Autodesk Inventor part; units mm, degrees
ref_plane "YZ Plane" through (0, 0, 0) normal (1, 0, 0) x (0, 1, 0)
ref_plane "XZ Plane" through (0, 0, 0) normal (0, 1, 0) x (-1, 0, 0)
ref_plane "XY Plane" through (0, 0, 0) normal (0, 0, 1) x (1, 0, 0)
sketch "Sketch1" plane through (0, 0, 0) normal (0, 0, 1) x (1, 0, 0)
  line L0 (0, 0) -> (30, 0)
  line L1 (30, 0) -> (30, 12.5)
  line L2 (30, 12.5) -> (0, 12.5)
  line L3 (0, 12.5) -> (0, 0)
  circle A0 centre (15, 0) radius 8
  point P0 (7, 0)
  point P1 (23, 0)
  dimension "d0" = 30
  dimension "d1" = 12.5
  dimension "d2" = 16
extrude "Extrusion1" add sketch "Sketch1" along normal mid plane 16 contours A0 L0 L3 L2 L1
sketch "Sketch2" plane through (0, 12.5, 8) normal (0, 1, 0) x (1, 0, 0)
  line L0 (0, 16) -> (0, 0)
  line L1 (30, 0) -> (0, 0)
  line L2 (30, 16) -> (30, 0)
  line L3 (0, 16) -> (30, 16)
  line L4 (23, 0) -> (7, 0)
  line L5 (15, 0) -> (15, 16)
  line L6 (0, 8) -> (30, 8)
  line L7 (2.5, 3) -> (27.5, 3)
  line L8 (27.5, 3) -> (27.5, 13)
  line L9 (27.5, 13) -> (2.5, 13)
  line L10 (2.5, 13) -> (2.5, 3)
  point P0 (15, 8)
  dimension "d5" = 25
  dimension "d6" = 10
hole "Hole1" at (2.5, 12.5, 5) at (2.5, 12.5, -5) at (27.5, 12.5, -5) at (27.5, 12.5, 5) at (15, 12.5, 0) direction (0, -1, 0) diameter 3 end through all
fillet "Fillet1" radius 2 4 edges at (0, 6.25, 8) (30, 6.25, -8) (30, 6.25, 8) (0, 6.25, -8)
properties part number "base2" material "PVC-Piping"
Could you check a few things on this model? Use its own coordinates, in mm. Give positions to 0.01 mm unless a question says otherwise; leave off trailing zeros. Loops run counter-clockwise (first coordinate to the right, second up) from the corner with the lowest first, then second, coordinate; pieces in that order, holes last. Notation, with made-up numbers: M -8.75,70 L 11.25,70 A21 ccw 11.25,83 Z; hole C -3.75,-36.75 d2. An arc over 180 degrees is marked long. Answer as a JSON object with one key per item and string values.
Q1. If we mould it in two halves opening along X, with no side actions, what happens to faces 1 (the flat face through (3, 0, 0)), 2 (the cylindrical face through (0.57, 6.16, -7.4)), 3 (the cylindrical face through (26, 6, -5))? For each: pulls with the +X half, pulls with the -X half, needs draft (parallel to the pull), parting line crosses it, or undercut.
Values found:
{"face 1": "needs draft", "face 2": "pulls with the -X half", "face 3": "undercut"}
Q2. If I drill on probe 1 along Z at (x, y) = (27.5, 8); probe 2 along X at (y, z) = (5.25, -5); probe 3 along Z at (x, y) = (15, 9.3), over which ranges is the centre line in solid material (lowest first)? Write a range as [from, to].
Values found:
{"probe 1": "z = [-8, -6.5], [-3.5, 3.5], [6.5, 8]", "probe 2": "x = [0, 1], [4, 8.96], [21.04, 26], [29, 30]", "probe 3": "z = [-8, -1.5], [1.5, 8]"}
Q3. Suppose I cut it at C-C, the plane y = 4. List the corners of the cut face in (x, z) for me, plus the area to 3 significant figures.
Values found:
{"outline": "M 0,-6 A2 ccw 2,-8 L 8.07,-8 L 8.07,8 L 2,8 A2 ccw 0,6 Z; M 21.93,-8 L 28,-8 A2 ccw 30,-6 L 30,6 A2 ccw 28,8 L 21.93,8 Z; hole C 2.5,-5 d3; hole C 2.5,5 d3; hole C 27.5,-5 d3; hole C 27.5,5 d3", "area": "227 mm²"}
Q4. For P1, Ø2.5, axis at x = 2.5, z = 5, coming from the -Y side; P2, Ø4, axis at x = 18.5, z = -2, coming from the -Y side, each with a flat end and sliding along its axis, tell me the tip position at first contact or that it passes through.
Values found:
{"P1": "passes through", "P2": "stops at y = 5.81"}
Q5. Suppose I cut it at A-A, the plane x = 2.5. List the corners of the cut face in (y, z) for me.
Values found:
{"outline": "M 0,-8 L 12.5,-8 L 12.5,-6.5 L 0,-6.5 Z; M 0,-3.5 L 12.5,-3.5 L 12.5,3.5 L 0,3.5 Z; M 0,6.5 L 12.5,6.5 L 12.5,8 L 0,8 Z"}
Q6. Suppose I cut it at B-B, the plane z = 5. List the corners of the cut face in (x, y) for me, plus the area to 3 significant figures.
Values found:
{"outline": "M 0,0 L 1,0 L 1,12.5 L 0,12.5 Z; M 4,0 L 7,0 A8 cw 23,0 L 26,0 L 26,12.5 L 4,12.5 Z; M 29,0 L 30,0 L 30,12.5 L 29,12.5 Z", "area": "199 mm²"}
Q7. Suppose I cut it at D-D, the plane z = 0. List the corners of the cut face in (x, y) for me.
Values found:
{"outline": "M 0,0 L 7,0 A8 cw 13.5,7.86 L 13.5,12.5 L 0,12.5 Z; M 16.5,7.86 A8 cw 23,0 L 30,0 L 30,12.5 L 16.5,12.5 Z"}
